Design review of the part built by this model. Coordinates are the model's own, in mm. A direction names the side the tool comes from. Round coordinates to 2 decimals unless told otherwise and drop trailing zeros. Write each loop counter-clockwise with the first axis right and the second up, starting at its lowest first coordinate (ties: lowest second). Pieces come first, ordered by that corner, then holes. Notation, with made-up numbers: M -20.75,-23.75 L -11.75,-23.75 A18 cw -11.75,-19.75 Z; hole C 11.25,30.5 d6. An arc over 180 degrees is marked long. One line per question, with ' | ' between items. Start each with the question number.
Item 1: Insertion check: pin 1 Ø2 at (x, z) = (0, 1) entering from -Y; pin 2 Ø0.9 at (x, y) = (0.5, -1) entering from +Z; pin 3 Ø0.9 at (y, z) = (-2, 0) entering from -X. Each pin has a flat end and moves straight along its axis. Give the tip position at first contact, or say it passes through.
Item 2: Add section D-D, the plane x = -0.25. State the section outline as (y, z) points, and give its area (3 significant figures).
Item 3: Add section A-A, the plane y = -1.75. State the section outline as (x, z) points.
Item 4: Machinability: for faces 4 (the face through (0, -1, -4.25)), 5 (the face through (-4.9, -1, 0)), 6 (the face through (-2.9, -1, 0)), which of the approach directions +Z, -Z, +X, -X, +Y, -Y give a long, thin tool a straight path to every point of the face, cutting with its end or side? Answer none if there is none.
Item 5: For L1, parallel to Z at x = 0, y = -1.9; L2, parallel to X at y = -1.75, z = -0.75; L3, parallel to Y at x = -5.75, z = 0.5, list the stretches that pass through material, from the lowest coordinate up.
Item 6: Add section B-B, the plane x = -4.25. State the section outline as (y, z) points.
Item 7: Draft analysis for pull direction X (two halves, no side actions). For faces 1 (the face through (0, -1, 4.25)), 2 (the face through (4.9, -1, 0)), 3 (the face through (0, 0, 0)), state which applies: released by +X, released by -X, zero draft, split by the parting line, or undercut.
Item 8: Add section C-C, the plane z = -2.75. State the section outline as (x, y) points.
```python
from build123d import *

# Parameters (mm, degrees)
SKETCH1_W           = 20
SKETCH1_H           = 10
BOSS_EXTRUDE1_DEPTH = 3
SKETCH2_W           = 9.8
SKETCH2_H           = 8.5
SKETCH2_W_2         = 5.8
SKETCH2_H_2         = 4.5
BOSS_EXTRUDE2_DEPTH = 3


with BuildPart() as part:
    # Sketch1 → Boss-Extrude1 (new body)
    with BuildSketch(Plane(origin=(0, 0, 0), x_dir=(1, 0, 0), z_dir=(0, 1, 0))):
        Rectangle(SKETCH1_W, SKETCH1_H)
    extrude(amount=BOSS_EXTRUDE1_DEPTH)

    # Sketch2 → Boss-Extrude2 (add)
    with BuildSketch(Plane.XZ):
        Rectangle(SKETCH2_W, SKETCH2_H)
        Rectangle(SKETCH2_W_2, SKETCH2_H_2, mode=Mode.SUBTRACT)
    extrude(amount=BOSS_EXTRUDE2_DEPTH)


solid = part.part
```
Computed values:
1) pin 1: stops at y = 0 | pin 2: stops at z = 4.25 | pin 3: stops at x = -4.9
2) outline: M -3,-4.25 L 0,-4.25 L 0,-5 L 3,-5 L 3,5 L 0,5 L 0,4.25 L -3,4.25 L -3,2.25 L 0,2.25 L 0,-2.25 L -3,-2.25 Z | area: 42.0 mm^2
3) outline: M -4.9,-4.25 L 4.9,-4.25 L 4.9,4.25 L -4.9,4.25 Z; hole M -2.9,-2.25 L 2.9,-2.25 L 2.9,2.25 L -2.9,2.25 Z
4) face 4: -Z, +X, -X, -Y | face 5: +Z, -Z, -X, -Y | face 6: -Y
5) L1: z = -4.25 to -2.25, 2.25 to 4.25 | L2: x = -4.9 to -2.9, 2.9 to 4.9 | L3: y = 0 to 3
6) outline: M -3,-4.25 L 0,-4.25 L 0,-5 L 3,-5 L 3,5 L 0,5 L 0,4.25 L -3,4.25 Z
7) face 1: zero draft | face 2: released by +X | face 3: undercut
8) outline: M -10,0 L -4.9,0 L -4.9,-3 L 4.9,-3 L 4.9,0 L 10,0 L 10,3 L -10,3 Z
